Design review of the part built by this model. Coordinates are the model's own, in mm. A direction names the side the tool comes from. Give positions to 0.01 mm unless a question says otherwise; leave off trailing zeros. Write each loop counter-clockwise with the first axis right and the second up, starting at its lowest first coordinate (ties: lowest second). Pieces come first, ordered by that corner, then holes. Notation, with made-up numbers: (70.5, 39) -> (88.5, 39) arc R6 ccw to (88.5, 45) -> close; hole circle Ø11 at (-37.5, 36.25). An arc over 180 degrees is marked (long way). Write each question's results on one line, items separated by ' | '. Start each with the question number.
(1) Mouldability with a two-part tool opening along X and no side actions: class faces 1 (the face through (62.325, 86.665, 3.254)), 2 (the face through (30, 33.9, 3)), 3 (the face through (45.85, 62.77, 3.25)) as released by +X, released by -X, zero draft, split by the parting line, or undercut.
(2) Take a section at D-D (z = 2.5). Count the separate pieces of the cut face and the enclosed holes in it, plus the area to 3 significant figures.
(3) To check wall thickness, follow probe 1 along Y at (x, z) = (32.5, 1); probe 2 along Y at (x, z) = (21.36, 2); probe 3 along X at (y, z) = (50, 0.5). State the ranges of each line that lie inside material, in increasing order.
(4) For faces 4 (the face through (23, 73.95, 3)), 5 (the face through (50.19, 2, 3)), 6 (the face through (38, 39.535, 3)), 7 (the face through (5.78, -10, 3)), 8 (the face through (43, 33.9, 3)), list the 3-axis set-ups (+Z, -Z, +X, -X, +Y, -Y) from which the entire face can be reached by the end or side of a thin tool; tool diameter is ignored.
(5) Take a section at A-A (x = -14.5). State the section outline as (y, z) points, plus the area to 3 significant figures.
(6) Clearance check with a flat-ended pin moving along its axis: pin 1 (1 mm diameter, centred on y = 77, z = 3.5, fed in from -X). State where the tip first meets the part, or that it passes through.
(7) Take a section at B-B (y = 42). State the section outline as (x, z) points.
(8) Take a section at C-C (x = 3.43). State the section outline as (y, z) points, plus the area to 3 significant figures.
from build123d import *

# Parameters (mm, degrees)
MODEL_R             = 4.375
MODEL_R_2           = 2.9
MODEL_R_3           = 1.775
BOSS_EXTRUDE1_DEPTH = 6.6


with BuildPart() as part:
    # Model → Boss-Extrude1 (new body)
    with BuildSketch(Plane.XY):
        with BuildLine():
            Line((-24.79, -12.5), (-19.79, -17.5))
            Line((-19.79, -17.5), (-0.9195, -17.5))
            Line((-0.9195, -17.5), (1.0805, -15.5))
            Line((1.0805, -15.5), (1.0805, -4.8))
            ThreePointArc((1.0805, -4.8), (3.43, -2.4505), (5.7795, -4.8))
            Line((5.7795, -4.8), (5.7795, -15.5))
            Line((5.7795, -15.5), (7.7795, -17.5))
            Line((7.7795, -17.5), (45.19, -17.5))
            Line((45.19, -17.5), (50.19, -12.5))
            Line((50.19, -12.5), (50.19, 16.555))
            Line((50.19, 16.555), (55.19, 21.555))
            Line((55.19, 21.555), (59.79, 21.555))
            Line((59.79, 21.555), (64.79, 26.555))
            Line((64.79, 26.555), (64.79, 84.19991216))
            Line((64.79, 84.19991216), (59.79, 89.19991216))
            Line((59.79, 89.19991216), (24.79, 89.19991216))
            Line((24.79, 89.19991216), (24.79, 80.500006241))
            Line((24.79, 80.500006241), (35.79, 80.500006241))
            Line((35.79, 80.500006241), (35.79, 82.085006241))
            ThreePointArc((35.79, 82.085006241), (35.936446609, 82.438559632), (36.29, 82.585006241))
            Line((36.29, 82.585006241), (40.29, 82.585006241))
            ThreePointArc((40.29, 82.585006241), (40.643553391, 82.438559632), (40.79, 82.085006241))
            Line((40.79, 82.085006241), (40.79, 80.500006241))
            Line((40.79, 80.500006241), (45.29, 80.500006241))
            ThreePointArc((45.29, 80.500006241), (45.643553391, 80.353559632), (45.79, 80.000006241))
            Line((45.79, 80.000006241), (45.79, 77.450006241))
            ThreePointArc((45.79, 77.450006241), (45.643553391, 77.09645285), (45.29, 76.950006241))
            Line((45.29, 76.950006241), (40.79, 76.950006241))
            Line((40.79, 76.950006241), (40.79, 75.365006241))
            ThreePointArc((40.79, 75.365006241), (40.643553391, 75.01145285), (40.29, 74.865006241))
            Line((40.29, 74.865006241), (36.29, 74.865006241))
            ThreePointArc((36.29, 74.865006241), (35.936446609, 75.01145285), (35.79, 75.365006241))
            Line((35.79, 75.365006241), (35.79, 76.950006241))
            Line((35.79, 76.950006241), (24.79, 76.950006241))
            Line((24.79, 76.950006241), (24.79, 73.950006241))
            Line((24.79, 73.950006241), (20.79, 73.950006241))
            ThreePointArc((20.79, 73.950006241), (19.022233047, 73.217773194), (18.29, 71.450006241))
            Line((18.29, 71.450006241), (18.29, 47.950006241))
            ThreePointArc((18.29, 47.950006241), (19.022233047, 46.182239288), (20.79, 45.450006241))
            Line((20.79, 45.450006241), (24.79, 45.450006241))
            Line((24.79, 45.450006241), (24.79, 37.450006241))
            Line((24.79, 37.450006241), (35.79, 37.450006241))
            Line((35.79, 37.450006241), (35.79, 39.035006241))
            ThreePointArc((35.79, 39.035006241), (35.936446609, 39.388559632), (36.29, 39.535006241))
            Line((36.29, 39.535006241), (40.29, 39.535006241))
            ThreePointArc((40.29, 39.535006241), (40.643553391, 39.388559632), (40.79, 39.035006241))
            Line((40.79, 39.035006241), (40.79, 37.450006241))
            Line((40.79, 37.450006241), (45.29, 37.450006241))
            ThreePointArc((45.29, 37.450006241), (45.643553391, 37.303559632), (45.79, 36.950006241))
            Line((45.79, 36.950006241), (45.79, 34.400006241))
            ThreePointArc((45.79, 34.400006241), (45.643553391, 34.04645285), (45.29, 33.900006241))
            Line((45.29, 33.900006241), (40.79, 33.900006241))
            Line((40.79, 33.900006241), (40.79, 32.315006241))
            ThreePointArc((40.79, 32.315006241), (40.643553391, 31.96145285), (40.29, 31.815006241))
            Line((40.29, 31.815006241), (36.29, 31.815006241))
            ThreePointArc((36.29, 31.815006241), (35.936446609, 31.96145285), (35.79, 32.315006241))
            Line((35.79, 32.315006241), (35.79, 33.900006241))
            Line((35.79, 33.900006241), (24.79, 33.900006241))
            Line((24.79, 33.900006241), (24.79, 17.5))
            Line((24.79, 17.5), (-19.79, 17.5))
            Line((-19.79, 17.5), (-24.79, 12.5))
            Line((-24.79, 12.5), (-24.79, -12.5))
        make_face()
        with Locations((49.071999999, 59.812938251)):
            Circle(MODEL_R, mode=Mode.SUBTRACT)
        with Locations((57.621173682, 65.321162043)):
            Circle(MODEL_R_2, mode=Mode.SUBTRACT)
        with Locations((40.027151425, 64.462627946)):
            Circle(MODEL_R_2, mode=Mode.SUBTRACT)
        with Locations((49.567674891, 49.655024765)):
            Circle(MODEL_R_2, mode=Mode.SUBTRACT)
        with Locations((-14.5, -3.025)):
            Circle(MODEL_R_3, mode=Mode.SUBTRACT)
        with Locations((21.36, -3.025)):
            Circle(MODEL_R_3, mode=Mode.SUBTRACT)
    extrude(amount=BOSS_EXTRUDE1_DEPTH)


solid = part.part
Report:
1) face 1: released by +X | face 2: zero draft | face 3: undercut
2) separate pieces: 1 | enclosed holes: 6 | area: 5,140 mm2
3) probe 1: -17.5 to 33.9, 37.45 to 76.95, 80.5 to 89.2 | probe 2: -17.5 to -4.8, -1.25 to 17.5, 45.45 to 73.95 | probe 3: 18.29 to 46.69, 52.45 to 64.79
4) face 4: +Z, -Z, -X, +Y | face 5: +Z, -Z, +X, -Y | face 6: +Z, -Z | face 7: +Z, -Z, -Y | face 8: +Z, -Z, -X
5) outline: (-17.5, 0) -> (-4.8, 0) -> (-4.8, 6.6) -> (-17.5, 6.6) -> close; (-1.25, 0) -> (17.5, 0) -> (17.5, 6.6) -> (-1.25, 6.6) -> close | area: 208 mm2
6) pin 1: x = 24.79
7) outline: (24.79, 0) -> (64.79, 0) -> (64.79, 6.6) -> (24.79, 6.6) -> close
8) outline: (-2.45, 0) -> (17.5, 0) -> (17.5, 6.6) -> (-2.45, 6.6) -> close | area: 132 mm2
